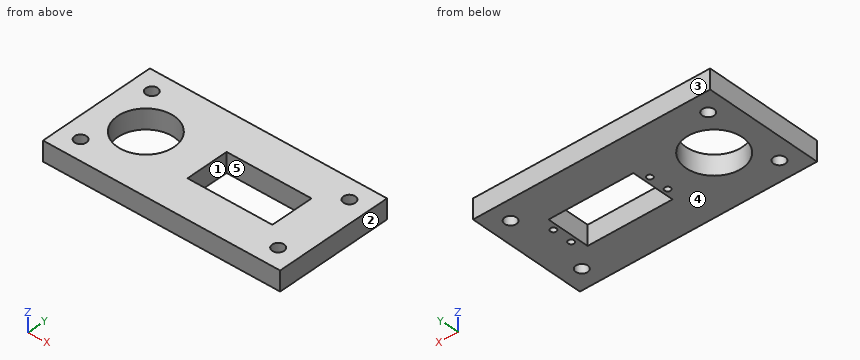
from build123d import *

# Parameters (mm, degrees)
CROQUIS1_W              = 120
CROQUIS1_H              = 60
SALIENTE_EXTRUIR1_DEPTH = 10
CROQUIS2_R              = 14.29
CROQUIS2_R_2            = 4.5
CORTAR_EXTRUIR1_DEPTH   = 68.823299831
CROQUIS3_W              = 42.957247878
CROQUIS3_H              = 21.957247878
CORTAR_EXTRUIR2_DEPTH   = 68.823299831
CROQUIS4_R              = 1.5
CORTAR_EXTRUIR3_DEPTH   = 8
CROQUIS5_W              = 40
CROQUIS5_H              = 60
SALIENTE_EXTRUIR2_DEPTH = 10
CROQUIS6_R              = 14.29
CORTAR_EXTRUIR4_DEPTH   = 105.880884817
CROQUIS7_W              = 40
CROQUIS7_H              = 60
CORTAR_EXTRUIR5_DEPTH   = 105.880884817
CROQUIS8_R              = 3
CORTAR_EXTRUIR6_DEPTH   = 68.823299831


with BuildPart() as part:
    # Croquis1 → Saliente-Extruir1 (new body)
    with BuildSketch(Plane.XY):
        Rectangle(CROQUIS1_W, CROQUIS1_H)
    extrude(amount=SALIENTE_EXTRUIR1_DEPTH)

    # Croquis2 → Cortar-Extruir1 (cut, through all)
    with BuildSketch(Plane.XY.offset(10)):
        with Locations((-35, 0)):
            Circle(CROQUIS2_R)
        with Locations((6.9608, 0)):
            Circle(CROQUIS2_R_2)
    extrude(amount=-CORTAR_EXTRUIR1_DEPTH, mode=Mode.SUBTRACT)

    # Croquis3 → Cortar-Extruir2 (cut, through all)
    with BuildSketch(Plane(origin=(0, 0, 0), x_dir=(-1, 0, 0), z_dir=(0, 0, -1))):
        with Locations((-17.4608, 0)):
            Rectangle(CROQUIS3_W, CROQUIS3_H)
    extrude(amount=-CORTAR_EXTRUIR2_DEPTH, mode=Mode.SUBTRACT)

    # Croquis4 → Cortar-Extruir3 (cut)
    with BuildSketch(Plane(origin=(0, 0, 0), x_dir=(-1, 0, 0), z_dir=(0, 0, -1))):
        with Locations((-41.8608, 5)):
            Circle(CROQUIS4_R)
        with Locations((6.9392, 5)):
            Circle(CROQUIS4_R)
        with Locations((6.9392, -5)):
            Circle(CROQUIS4_R)
        with Locations((-41.8608, -5)):
            Circle(CROQUIS4_R)
    extrude(amount=-CORTAR_EXTRUIR3_DEPTH, mode=Mode.SUBTRACT)

    # Croquis5 → Saliente-Extruir2 (add, through all)
    with BuildSketch(Plane.XY.offset(10)):
        with Locations((-80, 0)):
            Rectangle(CROQUIS5_W, CROQUIS5_H)
    extrude(amount=-SALIENTE_EXTRUIR2_DEPTH)

    # Croquis6 → Cortar-Extruir4 (cut, through all)
    with BuildSketch(Plane.XY.offset(10)):
        with Locations((-78.2308, 0)):
            Circle(CROQUIS6_R)
    extrude(amount=-CORTAR_EXTRUIR4_DEPTH, mode=Mode.SUBTRACT)

    # Croquis7 → Cortar-Extruir5 (cut, through all)
    with BuildSketch(Plane.XY.offset(10)):
        with Locations((-80, 0)):
            Rectangle(CROQUIS7_W, CROQUIS7_H)
    extrude(amount=-CORTAR_EXTRUIR5_DEPTH, mode=Mode.SUBTRACT)

    # Croquis8 → Cortar-Extruir6 (cut, through all)
    with BuildSketch(Plane(origin=(0, 0, 0), x_dir=(-1, 0, 0), z_dir=(0, 0, -1))):
        with Locations((-50, 20)):
            Circle(CROQUIS8_R)
        with Locations((50, 20)):
            Circle(CROQUIS8_R)
        with Locations((50, -20)):
            Circle(CROQUIS8_R)
        with Locations((-50, -20)):
            Circle(CROQUIS8_R)
    extrude(amount=-CORTAR_EXTRUIR6_DEPTH, mode=Mode.SUBTRACT)


solid = part.part
Here's how the part is built. I have some questions about the finished solid (model axes, mm). Face numbers are marked on the shaded views. A direction names the side the tool comes from. Coordinates: 2 decimals unless noted, no trailing zeros. Loops run counter-clockwise (first coordinate to the right, second up) from the corner with the lowest first, then second, coordinate; pieces in that order, holes last.
1. For the marked faces 1 and 2, which set-ups out of +Z, -Z, +X, -X, +Y, -Y let a thin tool reach every point of the face, with its end or its side?
2. I need wall thicknesses on L1, parallel to Y at x = 50, z = 3.75; L2, parallel to Y at x = -35, z = 4.25; L3, parallel to X at y = -7.5, z = 3.75. Which ranges of each line are inside material? Lowest first, please.
3. Imagine slicing it at B-B, the plane x = 18.5. Please give me the cut outline in (y, z), and give its area (3 significant figures).
4. For P1, Ø3.5, axis at x = -6, y = -5.5, coming from the -Z side, with a flat end and sliding along its axis, tell me the tip position at first contact or that it passes through.
5. Imagine slicing it at D-D, the plane x = 50. Please give me the cut outline in (y, z), and give its area (3 significant figures).
6. Imagine slicing it at A-A, the plane y = 0. Please give me the cut outline in (x, z), and give its area (3 significant figures).
7. Imagine slicing it at C-C, the plane z = 6.5. Count the separate pieces of the cut face and the enclosed holes in it, and give its area (3 significant figures).
8. If we mould it in two halves opening along Y, with no side actions, what happens to the marked faces 3, 4 and 5? For each: pulls with the +Y half, pulls with the -Y half, needs draft (parallel to the pull), parting line crosses it, or undercut.
Taken from the geometry:
1. face 1: +Z, -Z
1. face 2: +Z, -Z, +X, +Y, -Y
2. L1: y = -30 to -23, -17 to 17, 23 to 30
2. L2: y = -30 to -14.29, 14.29 to 30
2. L3: x = -60 to -47.16, -22.84 to -4.02, 38.94 to 60
3. outline: (-30, 0) - (-10.98, 0) - (-10.98, 10) - (-30, 10) - close; (10.98, 0) - (30, 0) - (30, 10) - (10.98, 10) - close
3. area: 380 mm2
4. P1: stops at z = 0
5. outline: (-30, 0) - (-23, 0) - (-23, 10) - (-30, 10) - close; (-17, 0) - (17, 0) - (17, 10) - (-17, 10) - close; (23, 0) - (30, 0) - (30, 10) - (23, 10) - close
5. area: 480 mm2
6. outline: (-60, 0) - (-49.29, 0) - (-49.29, 10) - (-60, 10) - close; (-20.71, 0) - (-4.02, 0) - (-4.02, 10) - (-20.71, 10) - close; (38.94, 0) - (60, 0) - (60, 10) - (38.94, 10) - close
6. area: 485 mm2
7. separate pieces: 1
7. enclosed holes: 10
7. area: 5,470 mm2
8. face 3: pulls with the +Y half
8. face 4: needs draft
8. face 5: undercut
